For this review, take the finished solid that the model builds, in its own axes (mm). Coordinates: 2 decimals unless noted, no trailing zeros. Loops run counter-clockwise (first coordinate to the right, second up) from the corner with the lowest first, then second, coordinate; pieces in that order, holes last. Notation, with made-up numbers: M 49,11.25 L 72,11.25 A24 ccw 72,34.25 Z; hole C 3,-13.5 d11. An arc over 180 degrees is marked long. Put each result on its own line as item: value.
Autodesk Inventor part; units mm, degrees
ref_plane "YZ Plane" through (0, 0, 0) normal (1, 0, 0) x (0, 1, 0)
ref_plane "XZ Plane" through (0, 0, 0) normal (0, 1, 0) x (-1, 0, 0)
ref_plane "XY Plane" through (0, 0, 0) normal (0, 0, 1) x (1, 0, 0)
sketch "Sketch1" plane through (0, 0, 0) normal (0, 0, 1) x (1, 0, 0)
  line L0 (0, 3.7) -> (-2.6393, 3.7)
  line L1 (-2.6393, 3.7) -> (-5.5, 6.5607)
  line L2 (-5.5, 6.5607) -> (-5.5, 8.2)
  line L3 (-5.5, 8.2) -> (-3.395, 8.2)
  line L4 (-3.395, 8.2) -> (-3.395, 10)
  line L5 (-3.395, 10) -> (-10, 10)
  line L6 (-10, 10) -> (-10, 3.395)
  line L7 (-10, 3.395) -> (-8.2, 3.395)
  line L8 (-8.2, 3.395) -> (-8.2, 5.5)
  line L9 (-8.2, 5.5) -> (-6.5607, 5.5)
  line L10 (-6.5607, 5.5) -> (-3.7, 2.6393)
  line L11 (-3.7, 2.6393) -> (-3.7, 0)
  line L12 (0, 0) -> (-10, 10) construction
  circle A0 centre (0, 0) radius 2.3
  line L13 (-22.6601, 0) -> (65.9605, 0)
  line L14 (-3.7, 0) -> (0, 0)
  line L15 (0, 0) -> (0, 3.7)
  line L16 (11.2521, 18.9743) -> (53.3004, 18.9743) construction
  line L17 (53.3004, 18.9743) -> (53.3004, -5.624) construction
  line L18 (53.3004, -5.624) -> (11.2521, -5.624) construction
  line L19 (11.2521, -5.624) -> (11.2521, 18.9743) construction
  point P0 (-2.3, 0)
  point P1 (0, 2.3)
  dimension "d0" = 1.5
  dimension "d6" = 6.3
  dimension "d9" = 4.6
  dimension "d18" = 135
  dimension "d22" = 20
  dimension "d34" = 11
  dimension "d35" = 6.79
  dimension "d36" = 1.8
extrude "Extrusion1" add sketch "Sketch1" along normal mid plane 200 contours L15 A0 L13 L11 L10 L9 L8 L7 L6 L5 L4 L3 L2 L1 L0
pattern_circular "Circular Pattern1" count 4 over 360 about axis through (0, 0, -10) along (0, 0, 1) of "Extrusion1"
chamfer "Chamfer1" distance 1.185 angle 45 8 edges at (-3.395, 10, 0) (3.395, 10, 0) (10, 3.395, 0) (10, -3.395, 0) (3.395, -10, 0) (-3.395, -10, 0) (-10, -3.395, 0) (-10, 3.395, 0)
fillet "Fillet1" radius 1.5 4 edges at (-10, 10, 0) (10, 10, 0) (-10, -10, 0) (10, -10, 0)
properties part number "2020aluminum_extrusion_black" material "Aluminum 6061"
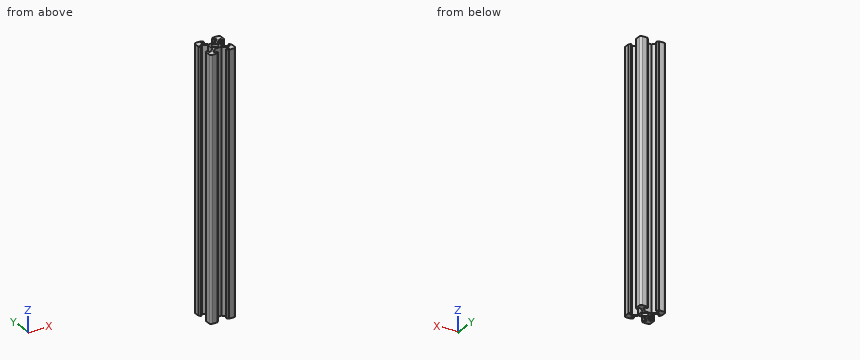
(1) For pin 1 (3 mm diameter, centred on x = -2.5, z = -29.5, fed in from -Y); pin 2 (3 mm diameter, centred on x = 1, z = 17, fed in from -Y); pin 3 (1.6 mm diameter, centred on x = 0, z = -16.5, fed in from +Y), all flat-tipped, find the tip position at first contact; note any pin that passes through.
Determined:
pin 1: stops at y = -9.42
pin 2: stops at y = -3.7
pin 3: stops at y = 3.7
(2) Wall thickness on line 1 along Y through (x, z) = (4.25, 57); line 2 along Y through (x, z) = (0, -26): over which ranges is each line inside the solid? List them lowest first. Write a range as [from, to].
Determined:
line 1: y = [-9.67, -8.2], [-5.31, -3.19], [3.19, 5.31], [8.2, 9.67]
line 2: y = [-3.7, -2.3], [2.3, 3.7]
(3) Add section A-A (y = 0). Write out the cut boundary in (x, z), plus the area to 3 significant figures.
Determined:
outline: M -3.7,-100 L -2.3,-100 L -2.3,100 L -3.7,100 Z; M 2.3,-100 L 3.7,-100 L 3.7,100 L 2.3,100 Z
area: 560 mm^2
